CAD build for the part. Positions are in the model's coordinates, mm. Face numbers are marked on the shaded views. A direction names the side the tool comes from. Coordinates: 2 decimals unless noted, no trailing zeros. Loops run counter-clockwise (first coordinate to the right, second up) from the corner with the lowest first, then second, coordinate; pieces in that order, holes last. Notation, with made-up numbers: (35, 76.25) - (77, 76.25) arc R16 cw to (77, 81.25) - close; hole circle Ø4 at (67.5, 60). An arc over 180 degrees is marked (long way). Put each result on its own line as item: value.
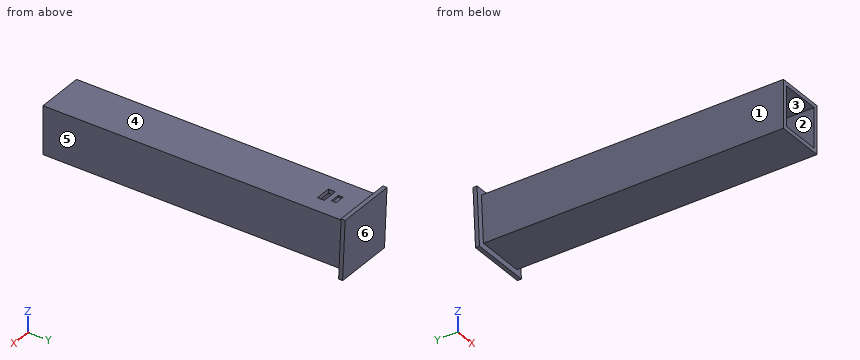
```python
from build123d import *

# Parameters (mm, degrees)
SKETCH_1_W          = 240
SKETCH_1_H          = 240
SKETCH_1_W_2        = 200
SKETCH_1_H_2        = 200
EXTRUDE_1_DEPTH     = 1500
SKETCH_2_W          = 78
SKETCH_2_H          = 34.5
CUT_EXTRUDE_1_DEPTH = 20
EXTRUDE_2_DEPTH     = 240
SKETCH_4_W          = 300
SKETCH_4_H          = 300.208242989
EXTRUDE_3_DEPTH     = 20
SKETCH_6_W          = 49
SKETCH_6_H          = 24
CUT_EXTRUDE_3_DEPTH = 10


with BuildPart() as part:
    # Эскиз1 → Бобышка-Вытянуть1 (new body)
    with BuildSketch(Plane(origin=(0, 0, 0), x_dir=(1, 0, 0), z_dir=(0, 1, 0))):
        with Locations((-163.322789272, 28.35162174)):
            Rectangle(SKETCH_1_W, SKETCH_1_H)
        with Locations((-163.322789272, 28.35162174)):
            Rectangle(SKETCH_1_W_2, SKETCH_1_H_2, mode=Mode.SUBTRACT)
    extrude(amount=EXTRUDE_1_DEPTH)

    # Эскиз2 → Вырез-Вытянуть1 (cut)
    with BuildSketch(Plane.XY.offset(91.64837826)):
        with Locations((-163.322789272, 1332.75)):
            Rectangle(SKETCH_2_W, SKETCH_2_H)
    extrude(amount=-CUT_EXTRUDE_1_DEPTH, mode=Mode.SUBTRACT)

    # Эскиз3 → Бобышка-Вытянуть2 (add)
    with BuildSketch(Plane.ZY.offset(283.322789272)):
        Polygon((-148.35162174, 1500), (91.64837826, 1500), (91.64837826, 1510), align=None)
    extrude(amount=-EXTRUDE_2_DEPTH)

    # Эскиз4 → Бобышка-Вытянуть3 (add)
    with BuildSketch(Plane(origin=(0, 1503.570951338, -62.648789639), x_dir=(1, 0, 0), z_dir=(0, 0.999133073092352, -0.041630544712181396))):
        with Locations((-163.322789272, -34.326926836)):
            Rectangle(SKETCH_4_W, SKETCH_4_H)
    extrude(amount=EXTRUDE_3_DEPTH)

    # Эскиз6 → Вырез-Вытянуть3 (cut)
    with BuildSketch(Plane.XY.offset(91.64837826)):
        with Locations((-163.322789272, 1387.5)):
            Rectangle(SKETCH_6_W, SKETCH_6_H)
    extrude(amount=-CUT_EXTRUDE_3_DEPTH, mode=Mode.SUBTRACT)


solid = part.part
```
Q1. Tool access for the marked faces 1 and 2: list every direction of +Z, -Z, +X, -X, +Y, -Y with a clear straight run to the whole face (end or side of a thin tool).
Determined:
face 1: +Z, -Z, -X, -Y
face 2: -Y
Q2. Slice it at B-B, the plane x = -163.5. Give the cut face in (y, z), then the cut area to 3 significant figures.
Determined:
outline: (0, -148.35) - (1500, -148.35) - (1498.75, -178.33) - (1518.73, -179.16) - (1531.23, 120.79) - (1511.25, 121.62) - (1510, 91.65) - (1399.5, 91.65) - (1399.5, 81.65) - (1375.5, 81.65) - (1375.5, 91.65) - (1350, 91.65) - (1350, 71.65) - (1500, 71.65) - (1500, -128.35) - (0, -128.35) - close; (0, 71.65) - (1315.5, 71.65) - (1315.5, 91.65) - (0, 91.65) - close
area: 66,300 mm2
Q3. Pin check, flat tips, straight feed: pin 1 Ø8 at (x, z) = (-170, 86) entering from +Y; pin 2 Ø5 at (x, y) = (-118.5, 1218.5) entering from +Z; pin 3 Ø2 at (x, y) = (-223.5, 443.5) entering from -Z. Stop position of each tip, or through.
Determined:
pin 1: y = 1529.95
pin 2: z = 91.65
pin 3: z = -148.35
Q4. Slice it at D-D, the plane z = -85. Give the cut face in (x, y), then the cut area to 3 significant figures.
Determined:
outline: (-313.32, 1502.64) - (-283.32, 1502.64) - (-283.32, 0) - (-263.32, 0) - (-263.32, 1500) - (-63.32, 1500) - (-63.32, 0) - (-43.32, 0) - (-43.32, 1502.64) - (-13.32, 1502.64) - (-13.32, 1522.66) - (-313.32, 1522.66) - close
area: 66,600 mm2
Q5. Mould opens along Z. For the marked faces 3, 4, 5 and 6 say: +Z half, -Z half, draft (parallel to the pull), parting line (faces both ways), or undercut.
Determined:
face 3: undercut
face 4: +Z half
face 5: draft
face 6: -Z half
Q6. Wall check: L1, parallel to X at y = 1454, z = -100.5; L2, parallel to Z at x = -153, y = 140.5; L3, parallel to X at y = 896, z = 76. Give the ranges that are in metal, low to high. Write a range as from..to.
Determined:
L1: -283.32..-263.32, -63.32..-43.32
L2: -148.35..-128.35, 71.65..91.65
L3: -283.32..-43.32
Q7. Slice it at C-C, the plane x = -232. Give the cut face in (y, z), then the cut area to 3 significant figures.
Determined:
outline: (0, -148.35) - (1500, -148.35) - (1498.75, -178.33) - (1518.73, -179.16) - (1531.23, 120.79) - (1511.25, 121.62) - (1510, 91.65) - (0, 91.65) - (0, 71.65) - (1500, 71.65) - (1500, -128.35) - (0, -128.35) - close
area: 67,200 mm2
Q8. Slice it at A-A, the plane y = 764.5. Give the cut face in (x, z).
Determined:
outline: (-283.32, -148.35) - (-43.32, -148.35) - (-43.32, 91.65) - (-283.32, 91.65) - close; hole (-263.32, -128.35) - (-63.32, -128.35) - (-63.32, 71.65) - (-263.32, 71.65) - close
